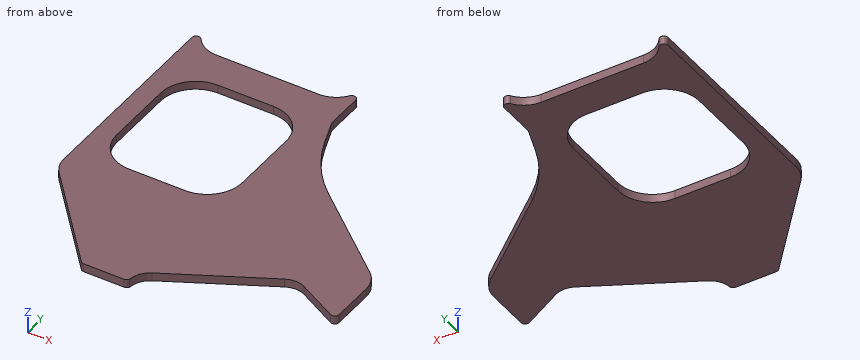
```python
from build123d import *

# Parameters (mm, degrees)
EXTRUDE1_DEPTH = 6


with BuildPart() as part:
    # Sketch1 → Extrude1 (new body)
    with BuildSketch(Plane.XY):
        with BuildLine():
            Line((-7.042073442, -3.744336867), (-78.042073442, -41.495706515))
            ThreePointArc((-78.042073442, -41.495706515), (-83.857509511, -47.014349285), (-86, -54.739920408))
            Line((-86, -54.739920408), (-86, -53))
            ThreePointArc((-86, -53), (-86.878679656, -55.121320344), (-89, -56))
            Line((-89, -56), (-117.936315897, -56))
            ThreePointArc((-117.936315897, -56), (-119.180395625, -55.729883813), (-120.200444638, -54.968177087))
            Line((-120.200444638, -54.968177087), (-179.594191604, 13.35651301))
            ThreePointArc((-179.594191604, 13.35651301), (-183.233443785, 19.473545965), (-184.5, 26.47769359))
            Line((-184.5, 26.47769359), (-184.5, 171.038518603))
            ThreePointArc((-184.5, 171.038518603), (-182.384651737, 173.905117861), (-179.02173913, 172.729146611))
            ThreePointArc((-179.02173913, 172.729146611), (-171.842990213, 166.316433225), (-162.5, 164))
            Line((-162.5, 164), (-89, 164))
            ThreePointArc((-89, 164), (-79.657009787, 166.316433225), (-72.47826087, 172.729146611))
            ThreePointArc((-72.47826087, 172.729146611), (-69.115348263, 173.905117861), (-67, 171.038518603))
            Line((-67, 171.038518603), (-67, 145.763269807))
            ThreePointArc((-67, 145.763269807), (-66.84807753, 144.02678803), (-66.396926208, 142.343068374))
            Line((-66.396926208, 142.343068374), (-60.19025019, 125.290366164))
            ThreePointArc((-60.19025019, 125.290366164), (-48.13619254, 102.134736861), (-30.49974908, 82.887936184))
            Line((-30.49974908, 82.887936184), (32.855752194, 29.726358433))
            ThreePointArc((32.855752194, 29.726358433), (38.126155741, 22.857834805), (40, 14.40546957))
            Line((40, 14.40546957), (40, -16.275538819))
            ThreePointArc((40, -16.275538819), (38.545114225, -18.847040722), (35.591585312, -18.924381598))
            Line((35.591585312, -18.924381598), (7.042073442, -3.744336867))
            ThreePointArc((7.042073442, -3.744336867), (0, -1.98855076), (-7.042073442, -3.744336867))
        make_face()
        with BuildLine():
            Line((-145.5, 139), (-105.5, 139))
            ThreePointArc((-105.5, 139), (-87.82233047, 131.67766953), (-80.5, 114))
            Line((-80.5, 114), (-80.5, 64))
            ThreePointArc((-80.5, 64), (-87.82233047, 46.32233047), (-105.5, 39))
            Line((-105.5, 39), (-145.5, 39))
            ThreePointArc((-145.5, 39), (-163.17766953, 46.32233047), (-170.5, 64))
            Line((-170.5, 64), (-170.5, 114))
            ThreePointArc((-170.5, 114), (-163.17766953, 131.67766953), (-145.5, 139))
        make_face(mode=Mode.SUBTRACT)
    extrude(amount=EXTRUDE1_DEPTH)


solid = part.part
```
Check sheet for the modelled part. Datum: model origin and axes. Units: mm. Coordinates: 2 decimals unless noted, no trailing zeros. Write each loop counter-clockwise with the first axis right and the second up, starting at its lowest first coordinate (ties: lowest second). Pieces come first, ordered by that corner, then holes. Notation, with made-up numbers: (64.25, 12.5) -> (109.25, 12.5) arc R17 ccw to (109.25, 39.5) -> close; hole circle Ø11 at (2.25, 68). An arc over 180 degrees is marked (long way). Use a Markdown table: item, result.
1. Scan lines: line 1 along X through (y, z) = (146.5, 4.15); line 2 along X through (y, z) = (-18, 5.4); line 3 along X through (y, z) = (100, 4.75). Record each from-to range of solid material in increasing order.
Reported:
| item | result |
|---|---|
| line 1 | x = -184.5 to -67 |
| line 2 | x = -152.34 to -33.85, 33.85 to 39.45 |
| line 3 | x = -184.5 to -170.5, -80.5 to -46.6 |
2. Sectioned sample at B-B (y = 68.5). Enter the section's corners in (x, z).
Reported:
| item | result |
|---|---|
| outline | (-184.5, 0) -> (-170.5, 0) -> (-170.5, 6) -> (-184.5, 6) -> close; (-80.5, 0) -> (-13.35, 0) -> (-13.35, 6) -> (-80.5, 6) -> close |
3. Sectioned sample at D-D (x = -13.5). Enter the section's corners in (y, z).
Reported:
| item | result |
|---|---|
| outline | (-7.18, 0) -> (68.62, 0) -> (68.62, 6) -> (-7.18, 6) -> close |
4. Go/stop test with flat-tipped pins: pin 1 Ø3 at (x, z) = (-141, 4) entering from -Y; pin 2 Ø0.5 at (y, z) = (-54.5, 3.5) entering from -X; pin 3 Ø1.5 at (x, z) = (-76, 3.5) entering from +Y; pin 4 Ø8 at (x, y) = (8, 36.5) entering from -Z. Record where each tip stops, or that it passes through.
Reported:
| item | result |
|---|---|
| pin 1 | stops at y = -32.77 |
| pin 2 | stops at x = -120.82 |
| pin 3 | stops at y = 169.48 |
| pin 4 | stops at z = 0 |
5. Sectioned sample at C-C (x = -141). Enter the section's corners in (y, z), plus the area to 3 significant figures.
Reported:
| item | result |
|---|---|
| outline | (-31.04, 0) -> (39, 0) -> (39, 6) -> (-31.04, 6) -> close; (139, 0) -> (164, 0) -> (164, 6) -> (139, 6) -> close |
| area | 570 mm2 |
